Verification items for the finished model (mm, model axes). Give positions to 0.01 mm unless a question says otherwise; leave off trailing zeros. Loops run counter-clockwise (first coordinate to the right, second up) from the corner with the lowest first, then second, coordinate; pieces in that order, holes last. Notation, with made-up numbers: (45, -28.75) - (94, -28.75) arc R28 ccw to (94, 8.25) - close; hole circle Ø8 at (27, 33.5). An arc over 180 degrees is marked (long way). One line per item, written item: value. Start each with the question number.
1. Scan lines: L1, parallel to Y at x = -10, z = 1.35; L2, parallel to X at y = -225, z = 1.1; L3, parallel to X at y = -188.5, z = 3.25. Record each from-to range of solid material in increasing order. Write a range as [from, to].
2. Sectioned sample at D-D (z = 5.5). Record the cut outline in (x, y), plus the area to 3 significant figures.
3. Sectioned sample at A-A (x = -10). Record the cut outline in (y, z).
4. Mould release check, pull along X, two halves, no side actions. Record for faces 1 (the flat face through (-2, -123, 11)), 2 (the cylindrical face through (-10.273, -227.082, 0.986)), 3 (the flat face through (-11, -123, 2)), 4 (the flat face through (0, -123, 10)): pulls with the +X half, pulls with the -X half, needs draft (parallel to the pull), parting line crosses it, or undercut.
5. Sectioned sample at C-C (y = -29). Record the cut outline in (x, z), plus the area to 3 significant figures.
6. Sectioned sample at B-B (y = -75). Record the cut outline in (x, z), plus the area to 3 significant figures.
7. Gauge pin test, flat ends, axial feed: pin 1 (5.5 mm diameter, centred on x = -10, y = -225, fed in from +Z); pin 2 (2.5 mm diameter, centred on x = -10, y = -75, fed in from -Z); pin 3 (2 mm diameter, centred on x = -10.5, y = -170.5, fed in from -Z). Record the tip position at first contact, or that the pin passes through.
from build123d import *

# Parameters (mm, degrees)
F1_DEPTH = 250
F2_R     = 2.1
F3_DEPTH = 25


with BuildPart() as f1:
    # F0 (on Front) → F1 (new body)
    with BuildSketch(Plane.XZ):
        with BuildLine():
            ThreePointArc((-0.5, 0), (-0.146447, 0.146447), (0, 0.5))
            Line((0, 0.5), (0, 19.5))
            ThreePointArc((0, 19.5), (-0.146447, 19.853553), (-0.5, 20))
            Line((-0.5, 20), (-1.5, 20))
            ThreePointArc((-1.5, 20), (-1.853553, 19.853553), (-2, 19.5))
            Line((-2, 19.5), (-2, 2.5))
            ThreePointArc((-2, 2.5), (-2.146447, 2.146447), (-2.5, 2))
            Line((-2.5, 2), (-19.5, 2))
            ThreePointArc((-19.5, 2), (-19.853553, 1.853553), (-20, 1.5))
            Line((-20, 1.5), (-20, 0.5))
            ThreePointArc((-20, 0.5), (-19.853553, 0.146447), (-19.5, 0))
            Line((-19.5, 0), (-0.5, 0))
        make_face()
    extrude(amount=F1_DEPTH)

    # F2 (on face) → F3 (cut)
    with BuildSketch(Plane(origin=(0, 0, 0), x_dir=(1, 0, 0), z_dir=(0, 0, -1))):
        with Locations((-10, 225)):
            Circle(F2_R)
        with Locations((-10, 150)):
            Circle(F2_R)
        with Locations((-10, 75)):
            Circle(F2_R)
        with Locations((-10, 0)):
            Circle(F2_R)
        with Locations((-10, -75)):
            Circle(F2_R)
    extrude(amount=-F3_DEPTH, mode=Mode.SUBTRACT)


solid = f1.part
Results are:
1. L1: y = [-250, -227.1], [-222.9, -152.1], [-147.9, -77.1], [-72.9, -2.1]
1. L2: x = [-20, -12.1], [-7.9, 0]
1. L3: x = [-2, 0]
2. outline: (-2, -250) - (0, -250) - (0, 0) - (-2, 0) - close
2. area: 500 mm^2
3. outline: (-250, 0) - (-227.1, 0) - (-227.1, 2) - (-250, 2) - close; (-222.9, 0) - (-152.1, 0) - (-152.1, 2) - (-222.9, 2) - close; (-147.9, 0) - (-77.1, 0) - (-77.1, 2) - (-147.9, 2) - close; (-72.9, 0) - (-2.1, 0) - (-2.1, 2) - (-72.9, 2) - close
4. face 1: pulls with the -X half
4. face 2: undercut
4. face 3: needs draft
4. face 4: pulls with the +X half
5. outline: (-20, 0.5) arc R0.5 ccw to (-19.5, 0) - (-0.5, 0) arc R0.5 ccw to (0, 0.5) - (0, 19.5) arc R0.5 ccw to (-0.5, 20) - (-1.5, 20) arc R0.5 ccw to (-2, 19.5) - (-2, 2.5) arc R0.5 cw to (-2.5, 2) - (-19.5, 2) arc R0.5 ccw to (-20, 1.5) - close
5. area: 75.8 mm^2
6. outline: (-20, 0.5) arc R0.5 ccw to (-19.5, 0) - (-12.1, 0) - (-12.1, 2) - (-19.5, 2) arc R0.5 ccw to (-20, 1.5) - close; (-7.9, 0) - (-0.5, 0) arc R0.5 ccw to (0, 0.5) - (0, 19.5) arc R0.5 ccw to (-0.5, 20) - (-1.5, 20) arc R0.5 ccw to (-2, 19.5) - (-2, 2.5) arc R0.5 cw to (-2.5, 2) - (-7.9, 2) - close
6. area: 67.4 mm^2
7. pin 1: stops at z = 2
7. pin 2: passes through
7. pin 3: stops at z = 0
